Here's how the part is built. I have some questions about the finished solid (model axes, mm). A direction names the side the tool comes from. Coordinates: 2 decimals unless noted, no trailing zeros. Write each loop counter-clockwise with the first axis right and the second up, starting at its lowest first coordinate (ties: lowest second). Pieces come first, ordered by that corner, then holes.
Item 1: If we section it at D-D (x = -24): Please give me the cut outline in (y, z).
Item 2: I'm going to push flat-ended pins straight in: pin 1 Ø0.8 at (x, z) = (11.5, 1.5) entering from -Y; pin 2 Ø0.8 at (y, z) = (-77, 1) entering from +X; pin 3 Ø10 at (x, y) = (-4, -71.5) entering from +Z. Where does each tip first touch, or does it pass through?
Item 3: If we section it at C-C (y = -31.75): Please give me the cut outline in (x, z) (3 decimals), then the cut area to 3 significant figures.
Item 4: If we section it at B-B (x = 3.5): Please give me the cut outline in (y, z).
Item 5: We'd pull the mould along Y, two halves only. Please class faces 1 (the face through (3, -53.86, 1)), 2 (the face through (-31.693, -35.167, 1.232)), 3 (the face through (3, -62.01, 1)): +Y half, -Y half, draft (parallel to the pull), parting line (faces both ways), or undercut.
Item 6: If I drill on line 1 (Y direction, x = 1.5, z = 0.7); line 2 (X direction, y = -54.5, z = 2.4); line 3 (X direction, y = -73, z = 2.05), over which ranges is the centre line in solid material (lowest first)?
Item 7: For faces 4 (the face through (-13.865, -55.699, 1.232)), 5 (the face through (-1, -25.4, 1)), 6 (the face through (-22.047, -75, 1)), which set-ups out of +Z, -Z, +X, -X, +Y, -Y let a thin tool reach every point of the face, with its end or its side?
Item 8: If we section it at A-A (z = 0.9): Please give me the cut outline in (x, y) (3 decimals), then the cut area to 3 significant figures.
Autodesk Inventor part; units mm, degrees
ref_plane "YZ Plane" through (0, 0, 0) normal (1, 0, 0) x (0, 1, 0)
ref_plane "XZ Plane" through (0, 0, 0) normal (0, 1, 0) x (-1, 0, 0)
ref_plane "XY Plane" through (0, 0, 0) normal (0, 0, 1) x (1, 0, 0)
ref_plane "Work Plane1" through (0, 0, 0) normal (0, 0, 1) x (1, 0, 0)
sketch "Sketch1" plane through (0, 0, 0) normal (0, 0, 1) x (1, 0, 0)
  line L0 (11.43, 0) -> (11.43, -63.5) construction
  line L1 (0, 0) -> (11.43, 0) construction
  line L2 (0, 0) -> (0, -63.5) construction
  line L3 (7.44, -34.7378) -> (0, -34.7378) construction
  circle A0 centre (5.715, -31.75) radius 1.7 construction
  line L4 (0, -63.5) -> (11.43, -63.5) construction
  circle A1 centre (5.715, -55.6597) radius 1.7 construction
  line L5 (21.59, -62.0097) -> (-15.6718, -62.0097)
  line L6 (-22.0218, -25.4) -> (21.59, -25.4)
  line L7 (21.59, -25.4) -> (21.59, -62.0097)
  line L8 (18.415, -31.75) -> (-12.065, -31.75) construction
  line L9 (18.415, -29.95) -> (-12.065, -29.95)
  line L10 (-12.065, -33.55) -> (18.415, -33.55)
  arc A2 (18.415, -33.55) -> (18.415, -29.95) centre (18.415, -31.75) ccw
  arc A3 (-12.065, -29.95) -> (-12.065, -33.55) centre (-12.065, -31.75) ccw
  line L11 (18.415, -55.6597) -> (-12.065, -55.6597) construction
  line L12 (18.415, -53.8597) -> (-12.065, -53.8597)
  line L13 (-12.065, -57.4597) -> (18.415, -57.4597)
  arc A4 (18.415, -57.4597) -> (18.415, -53.8597) centre (18.415, -55.6597) ccw
  arc A5 (-12.065, -53.8597) -> (-12.065, -57.4597) centre (-12.065, -55.6597) ccw
  circle A6 centre (-31.5722, -81.8048) radius 4.826
  arc A7 (-41.0972, -81.8048) -> (-22.0472, -81.8048) centre (-31.5722, -81.8048) ccw
  line L14 (-22.0218, -25.4) -> (-22.0218, -62.0097) construction
  line L15 (-41.0972, -81.8048) -> (-4.0676, -81.8048) construction
  line L16 (-41.0972, -44.6639) -> (-22.0218, -25.4)
  line L17 (-22.0472, -81.8048) -> (-22.0472, -68.3851)
  line L18 (-15.6718, -62.0097) -> (-22.0472, -68.3851)
  line L19 (-15.6718, -62.0097) -> (-6.6556, -62.0097) construction
  line L20 (21.59, -43.7048) -> (-43.6873, -43.7048) construction
  line L21 (21.59, -43.7048) -> (86.8673, -43.7048) construction
  line L22 (-41.0972, -81.8048) -> (-29.4827, -81.8048) construction
  line L23 (-41.0972, -81.8048) -> (-41.0972, -44.6639)
  line L24 (-41.0972, -81.8048) -> (-3.9563, -81.8048) construction
  point P0 (3.175, -31.75)
  point P1 (3.175, -55.6597)
extrude "Extrusion1" add sketch "Sketch1" along normal blind 2.5
properties part number "driven wheel arm angled"
Answer list:
1. outline: (-87.58, 0) - (-27.4, 0) - (-27.4, 2.5) - (-87.58, 2.5) - close
2. pin 1: stops at y = -62.01
2. pin 2: stops at x = -22.05
2. pin 3: passes through
3. outline: (-28.31, 0) - (-13.865, 0) - (-13.865, 2.5) - (-28.31, 2.5) - close; (20.215, 0) - (21.59, 0) - (21.59, 2.5) - (20.215, 2.5) - close
3. area: 39.5 mm2
4. outline: (-62.01, 0) - (-57.46, 0) - (-57.46, 2.5) - (-62.01, 2.5) - close; (-53.86, 0) - (-33.55, 0) - (-33.55, 2.5) - (-53.86, 2.5) - close; (-29.95, 0) - (-25.4, 0) - (-25.4, 2.5) - (-29.95, 2.5) - close
5. face 1: undercut
5. face 2: +Y half
5. face 3: -Y half
6. line 1: y = -62.01 to -57.46, -53.86 to -33.55, -29.95 to -25.4
6. line 2: x = -41.1 to -13.44, 19.79 to 21.59
6. line 3: x = -41.1 to -22.05
7. face 4: +Z, -Z
7. face 5: +Z, -Z, +X, -X, +Y
7. face 6: +Z, -Z, +X, -Y
8. outline: (-41.097, -81.805) arc R9.525 ccw to (-22.047, -81.805) - (-22.047, -68.385) - (-15.672, -62.01) - (21.59, -62.01) - (21.59, -25.4) - (-22.022, -25.4) - (-41.097, -44.664) - close; hole circle Ø9.652 at (-31.572, -81.805); hole (-12.065, -57.46) - (18.415, -57.46) arc R1.8 ccw to (18.415, -53.86) - (-12.065, -53.86) arc R1.8 ccw to start; hole (-12.065, -33.55) - (18.415, -33.55) arc R1.8 ccw to (18.415, -29.95) - (-12.065, -29.95) arc R1.8 ccw to start
8. area: 2,340 mm2
